Can you work these out from the model? Positions are in its coordinate system, mm. Face numbers are marked on the shaded views. A direction names the side the tool comes from. Give positions to 0.01 mm unless a question says otherwise; leave off trailing zeros. Order: outer loops, then holes, each group sorted by start corner. A loop starts at its lowest first (then second) coordinate and runs counter-clockwise, first axis right, second up. Notation, with made-up numbers: (41, -37.5) - (66, -37.5) arc R25 ccw to (66, -14.5) - close; hole circle Ø1 at (-11, 39.5). An arc over 180 degrees is marked (long way). Write each question's results on one line, items separated by ' | '. Start each with the question number.
from build123d import *

# Parameters (mm, degrees)
F0_R     = 1.5
F0_R_2   = 1.6
F1_DEPTH = 2.1
F2_SIZE  = 1.75
F4_DEPTH = 0.1


with BuildPart() as f1:
    # F0 (on Top) → F1 (new body)
    with BuildSketch(Plane.XY):
        with BuildLine():
            Line((8.508672, 13.55), (-8.508672, 13.55))
            ThreePointArc((-8.508672, 13.55), (-13.153482, 9.10966), (-15.676734, 3.2))
            Line((-15.676734, 3.2), (-12, 3.2))
            ThreePointArc((-12, 3.2), (-9.737258, 2.262742), (-8.8, 0))
            ThreePointArc((-8.8, 0), (-9.737258, -2.262742), (-12, -3.2))
            Line((-12, -3.2), (-15.676734, -3.2))
            ThreePointArc((-15.676734, -3.2), (-13.153482, -9.10966), (-8.508672, -13.55))
            Line((-8.508672, -13.55), (0, -13.55))
            Line((0, -13.55), (8.508672, -13.55))
            ThreePointArc((8.508672, -13.55), (16, 0), (8.508672, 13.55))
        make_face()
        with Locations((-4.75, -8.25)):
            Circle(F0_R, mode=Mode.SUBTRACT)
        with BuildLine():
            ThreePointArc((1.6, -9.5), (1.131371, -10.631371), (0, -11.1))
            ThreePointArc((0, -11.1), (-1.131371, -8.368629), (1.6, -9.5))
        make_face(mode=Mode.SUBTRACT)
        with Locations((4.75, -8.25)):
            Circle(F0_R, mode=Mode.SUBTRACT)
        with Locations((-4.75, 8.25)):
            Circle(F0_R, mode=Mode.SUBTRACT)
        with Locations((0, 9.5)):
            Circle(F0_R_2, mode=Mode.SUBTRACT)
        with Locations((4.75, 8.25)):
            Circle(F0_R, mode=Mode.SUBTRACT)
    extrude(amount=F1_DEPTH)

    # F2
    f2_edges = [f1.edges().sort_by_distance(p)[0] for p in [
        (-1.6, -9.5, 2.1),
        (-1.6, 9.5, 2.1),
    ]]
    chamfer(f2_edges, length=F2_SIZE)

    # F3 (on face) → F4 (join)
    with BuildSketch(Plane.XY.offset(2.1)):
        with BuildLine():
            ThreePointArc((-12, 4), (-11.530048, 3.972297), (-11.066605, 3.889573))
            Line((-11.066605, 3.889573), (-11.066605, 10.419705))
            ThreePointArc((-11.066605, 10.419705), (-13.259799, 7.430863), (-14.664242, 4))
            Line((-14.664242, 4), (-12, 4))
        make_face()
        with BuildLine():
            Line((-12, -4), (-14.664242, -4))
            ThreePointArc((-14.664242, -4), (-13.259799, -7.430863), (-11.066605, -10.419705))
            Line((-11.066605, -10.419705), (-11.066605, -3.889573))
            ThreePointArc((-11.066605, -3.889573), (-11.530048, -3.972297), (-12, -4))
        make_face()
    extrude(amount=F4_DEPTH)


solid = f1.part
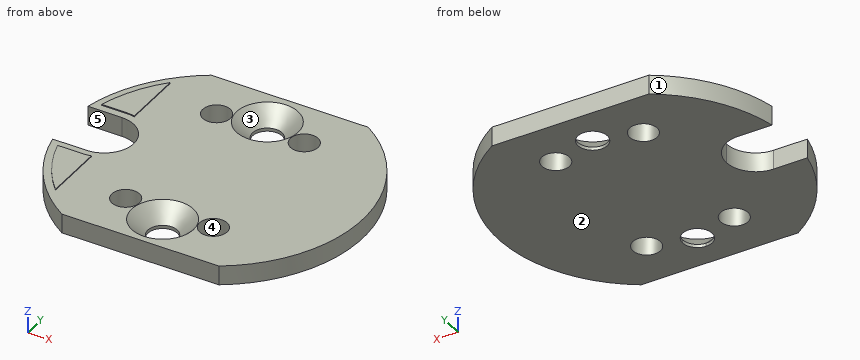
Q1. Thinking about a two-plate mould opening in X: for the marked faces 1, 2 and 3, which applies, released by +X, released by -X, zero draft, split by the parting line, or undercut?
Q2. If we section it at A-A (z = 1.4): Please give me the cut outline in (x, y), plus the area to 3 significant figures.
Q3. Will these pins go through, and if not, where does the flat tip stop? P1, Ø12, axis at x = 6.5, y = -2, coming from the +Z side; P2, Ø3.5, axis at x = 0, y = 9.5, coming from the +Z side.
Q4. If we section it at B-B (x = 4.75): Please give me the cut outline in (y, z).
Q5. If we section it at D-D (y = -8.25): State how many separate pieces and enclosed holes the cut face has, plus the area to 3 significant figures.
Q6. If I drill on probe 1 along Y at (x, z) = (0, 0.25); probe 2 along Y at (x, z) = (4.75, 1.4); probe 3 along X at (y, z) = (-8.75, 0.9), over which ranges is the centre line in solid material (lowest first)? Write a range as from..to.
Q7. If we section it at C-C (x = -13): Please give me the cut outline in (y, z), plus the area to 3 significant figures.
Q8. Which directions (+Z, -Z, +X, -X, +Y, -Y) give clear straight access to the entire face, cutting with the end or side of a thin tool? Please do the marked faces 4 and 5.
Findings below:
1) face 1: released by -X | face 2: zero draft | face 3: undercut
2) outline: (-15.68, -3.2) arc R16 ccw to (-8.51, -13.55) - (8.51, -13.55) arc R16 ccw to (8.51, 13.55) - (-8.51, 13.55) arc R16 ccw to (-15.68, 3.2) - (-12, 3.2) arc R3.2 cw to (-8.8, 0) arc R3.2 cw to (-12, -3.2) - close; hole circle Ø3 at (-4.75, -8.25); hole circle Ø3 at (-4.75, 8.25); hole circle Ø5.3 at (0, -9.5); hole circle Ø5.3 at (0, 9.5); hole circle Ø3 at (4.75, -8.25); hole circle Ø3 at (4.75, 8.25) | area: 634 mm2
3) P1: stops at z = 2.1 | P2: stops at z = 0.5
4) outline: (-13.55, 0) - (-9.75, 0) - (-9.75, 2.1) - (-13.55, 2.1) - close; (-6.75, 0) - (6.75, 0) - (6.75, 2.1) - (-6.75, 2.1) - close; (9.75, 0) - (13.55, 0) - (13.55, 2.1) - (9.75, 2.1) - close
5) separate pieces: 4 | enclosed holes: 0 | area: 37.1 mm2
6) probe 1: y = -13.55..-11.1, -7.9..7.9, 11.1..13.55 | probe 2: y = -13.55..-9.75, -6.75..6.75, 9.75..13.55 | probe 3: x = -13.4..-6.16, -3.34..-2.01, 2.01..3.34, 6.16..13.4
7) outline: (-9.33, 0) - (-3.2, 0) - (-3.2, 2.1) - (-4, 2.1) - (-4, 2.2) - (-7.88, 2.2) - (-7.88, 2.1) - (-9.33, 2.1) - close; (3.2, 0) - (9.33, 0) - (9.33, 2.1) - (7.88, 2.1) - (7.88, 2.2) - (4, 2.2) - (4, 2.1) - (3.2, 2.1) - close | area: 26.5 mm2
8) face 4: +Z, -Z | face 5: +Z, -Z, -X
